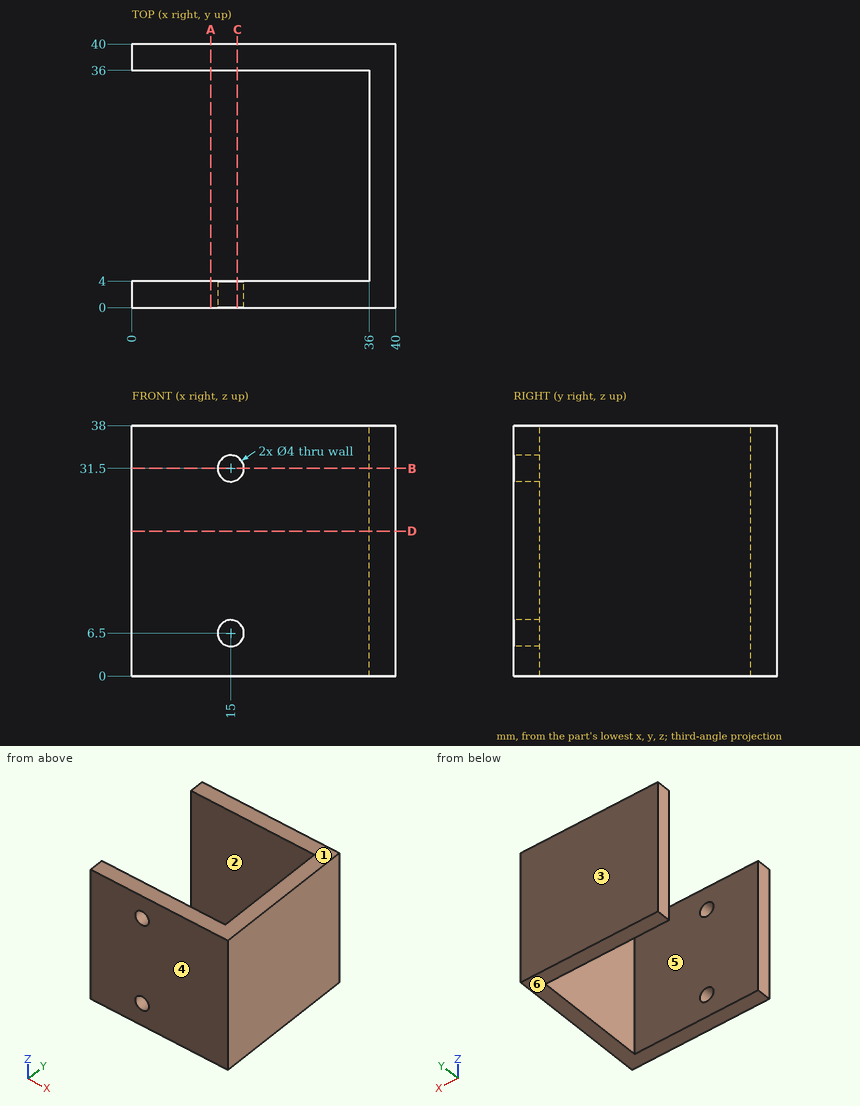
The drawing under review shows one solid part. Ordinate dimensions are in mm from its lowest x, y, z. A direction names the side the tool comes from. Coordinates: 2 decimals unless noted, no trailing zeros. Order: outer loops, then holes, each group sorted by start corner. A loop starts at its lowest first (then second) coordinate and runs counter-clockwise, first axis right, second up. Notation, with made-up numbers: (18, 5.25) -> (53, 5.25) arc R20 cw to (53, 12.25) -> close; hole circle Ø5 at (32.25, 59). An arc over 180 degrees is marked (long way). Return JSON: item names as keys, results as strings.
1. The part is to be moulded in two halves that separate along Y. For the marked faces 1, 2, 3 and 4, say which applies: +Y half, -Y half, draft (parallel to the pull), parting line (faces both ways), or undercut.
Answer block:
{"face 1": "draft", "face 2": "undercut", "face 3": "+Y half", "face 4": "-Y half"}
2. For line 1 (Z direction, x = 15, y = 1.05); line 2 (Y direction, x = 25.5, z = 3.5); line 3 (X direction, y = 24.5, z = 27), list the stretches that pass through material, from the lowest coordinate up. Write a range as from..to.
Answer block:
{"line 1": "0..4.5, 8.5..29.5, 33.5..38", "line 2": "0..4, 36..40", "line 3": "36..40"}
3. We need section B-B on z = 31.5. Write out the cut boundary in (x, y).
Answer block:
{"outline": "(0, 0) -> (13, 0) -> (13, 4) -> (0, 4) -> close; (0, 36) -> (36, 36) -> (36, 4) -> (17, 4) -> (17, 0) -> (40, 0) -> (40, 40) -> (0, 40) -> close"}
4. Machinability: for the marked faces 5 and 6, which of the approach directions +Z, -Z, +X, -X, +Y, -Y give a long, thin tool a straight path to every point of the face, cutting with its end or side? Answer none if there is none.
Answer block:
{"face 5": "+Z, -Z, -X", "face 6": "-Z, +X, -X, +Y, -Y"}
5. For pin 1 Ø4 at (y, z) = (17, 28.5) entering from -X, flat-tipped, find the tip position at first contact; note if it passes through.
Answer block:
{"pin 1": "x = 36"}
6. We need section C-C on x = 16. Write out the cut boundary in (y, z).
Answer block:
{"outline": "(0, 0) -> (4, 0) -> (4, 4.77) -> (0, 4.77) -> close; (0, 8.23) -> (4, 8.23) -> (4, 29.77) -> (0, 29.77) -> close; (0, 33.23) -> (4, 33.23) -> (4, 38) -> (0, 38) -> close; (36, 0) -> (40, 0) -> (40, 38) -> (36, 38) -> close"}
7. We need section A-A on x = 12. Write out the cut boundary in (y, z), and give its area (3 significant figures).
Answer block:
{"outline": "(0, 0) -> (4, 0) -> (4, 38) -> (0, 38) -> close; (36, 0) -> (40, 0) -> (40, 38) -> (36, 38) -> close", "area": "304 mm²"}
8. We need section D-D on z = 22. Write out the cut boundary in (x, y), and give its area (3 significant figures).
Answer block:
{"outline": "(0, 0) -> (40, 0) -> (40, 40) -> (0, 40) -> (0, 36) -> (36, 36) -> (36, 4) -> (0, 4) -> close", "area": "448 mm²"}
